from build123d import *

# Parameters (mm, degrees)
SKETCH1_W                                         = 279.4
SKETCH1_H                                         = 101.6
SKETCH1_R                                         = 2.15265
SKETCH1_W_2                                       = 6.604
SKETCH1_H_2                                       = 6.35
BOSS_EXTRUDE1_DEPTH                               = 6.604
CSK_FOR_8_FLAT_HEAD_SOCKET_CAP_SCREW1_D           = 4.3053
CSK_FOR_8_FLAT_HEAD_SOCKET_CAP_SCREW1_CSINK_D     = 9.1186
CSK_FOR_8_FLAT_HEAD_SOCKET_CAP_SCREW1_CSINK_ANGLE = 82


with BuildPart() as part:
    # Sketch1 → Boss-Extrude1 (new body)
    with BuildSketch(Plane(origin=(0, 0, 0), x_dir=(0, 0, -1), z_dir=(1, 0, 0))):
        with Locations((0, -50.8)):
            Rectangle(SKETCH1_W, SKETCH1_H)
        with Locations((-133.35, -24.8793)):
            Circle(SKETCH1_R, mode=Mode.SUBTRACT)
        with Locations((-133.35, -76.7207)):
            Circle(SKETCH1_R, mode=Mode.SUBTRACT)
        with Locations((133.35, -24.8793)):
            Circle(SKETCH1_R, mode=Mode.SUBTRACT)
        with Locations((133.35, -76.720700102)):
            Circle(SKETCH1_R, mode=Mode.SUBTRACT)
        with Locations((-133.35, -34.4043)):
            Rectangle(SKETCH1_W_2, SKETCH1_H_2, mode=Mode.SUBTRACT)
        with Locations((-133.35, -15.3543)):
            Rectangle(SKETCH1_W_2, SKETCH1_H_2, mode=Mode.SUBTRACT)
        with Locations((-133.35, -86.2457)):
            Rectangle(SKETCH1_W_2, SKETCH1_H_2, mode=Mode.SUBTRACT)
        with Locations((-133.35, -67.1957)):
            Rectangle(SKETCH1_W_2, SKETCH1_H_2, mode=Mode.SUBTRACT)
        with Locations((133.35, -15.3543)):
            Rectangle(SKETCH1_W_2, SKETCH1_H_2, mode=Mode.SUBTRACT)
        with Locations((133.35, -34.4043)):
            Rectangle(SKETCH1_W_2, SKETCH1_H_2, mode=Mode.SUBTRACT)
        with Locations((133.35, -67.195700102)):
            Rectangle(SKETCH1_W_2, SKETCH1_H_2, mode=Mode.SUBTRACT)
        with Locations((133.35, -86.245700102)):
            Rectangle(SKETCH1_W_2, SKETCH1_H_2, mode=Mode.SUBTRACT)
    extrude(amount=BOSS_EXTRUDE1_DEPTH)

    # CSK for #8 Flat Head Socket Cap Screw1 (through all)
    with Locations(Plane(origin=(6.604, 0, 0), x_dir=(0, 0, -1), z_dir=(1, 0, 0))):
        with Locations((-133.35, -24.8793), (-133.35, -76.7207), (133.35, -24.8793), (133.35, -76.720700102)):
            CounterSinkHole(CSK_FOR_8_FLAT_HEAD_SOCKET_CAP_SCREW1_D / 2, CSK_FOR_8_FLAT_HEAD_SOCKET_CAP_SCREW1_CSINK_D / 2, counter_sink_angle=CSK_FOR_8_FLAT_HEAD_SOCKET_CAP_SCREW1_CSINK_ANGLE)


solid = part.part
For this review, take the finished solid that the model builds, in its own axes (mm). A direction names the side the tool comes from. Round coordinates to 2 decimals unless told otherwise and drop trailing zeros. Put each result on its own line as item: value.
Q1. For probe 1 along Z at (x, y) = (5, -85); probe 2 along Z at (x, y) = (2, -23), list the stretches that pass through material, from the lowest coordinate up. Write a range as [from, to].
Check result:
probe 1: [-139.7, -136.65], [-130.05, 130.05], [136.65, 139.7]
probe 2: [-139.7, -134.4], [-132.3, 132.3], [134.4, 139.7]
Q2. Machinability: for faces 4 (the flat face through (3, -86, 130.048)), 5 (the flat face through (0, -50, 2)), which of the approach directions +Z, -Z, +X, -X, +Y, -Y give a long, thin tool a straight path to every point of the face, cutting with its end or side? Answer none if there is none.
Check result:
face 4: +X, -X
face 5: +Z, -Z, -X, +Y, -Y
Q3. Mouldability with a two-part tool opening along Y and no side actions: class faces 1 (the flat face through (3, -52, -139.7)), 2 (the flat face through (3, -101.6, 2)), 3 (the flat face through (3, -34, 136.652)) as pulls with the +Y half, pulls with the -Y half, needs draft (parallel to the pull), parting line crosses it, or undercut.
Check result:
face 1: needs draft
face 2: pulls with the -Y half
face 3: undercut
Q4. Insertion check: pin 1 Ø1 at (x, z) = (5, 28.5) entering from +Y; pin 2 Ø2.5 at (y, z) = (-76.72, 133.35) entering from +X. Each pin has a flat end and moves straight along its axis. Give the tip position at first contact, or say it passes through.
Check result:
pin 1: y = 0
pin 2: through
